For this review, take the finished solid that the model builds, in its own axes (mm). A direction names the side the tool comes from. Round coordinates to 2 decimals unless told otherwise and drop trailing zeros. Write each loop counter-clockwise with the first axis right and the second up, starting at its lowest first coordinate (ties: lowest second). Pieces come first, ordered by that corner, then holes. Notation, with made-up numbers: (25.5, 67.5) - (63.5, 67.5) arc R16 cw to (63.5, 77.5) - close; hole circle Ø7 at (27, 86.5). An arc over 180 degrees is marked (long way). Answer in a Markdown table with one row per item. Add a question column.
from build123d import *

# Parameters (mm, degrees)
SKETCH_1_R          = 15
EXTRUDE_2_DEPTH     = 28
SKETCH_3_R          = 1.5
CUT_EXTRUDE_3_DEPTH = 10
CUT_EXTRUDE_START   = -18
SKETCH_3_2_R        = 1.5
CUT_EXTRUDE_4_DEPTH = 10


with BuildPart() as part:
    # 草图1 → 凸台-拉伸2 (new body)
    with BuildSketch(Plane.XY):
        Circle(SKETCH_1_R)
    extrude(amount=EXTRUDE_2_DEPTH)

    # 草图3 → 切除-拉伸3 (cut)
    with BuildSketch(Plane.XY.offset(28)):
        Circle(SKETCH_3_R)
    extrude(amount=-CUT_EXTRUDE_3_DEPTH, mode=Mode.SUBTRACT)

    # 草图3<2> → 切除-拉伸4 (cut)
    with BuildSketch(Plane.XY.offset(28).offset(CUT_EXTRUDE_START)):
        Circle(SKETCH_3_2_R)
    extrude(amount=-CUT_EXTRUDE_4_DEPTH, mode=Mode.SUBTRACT)


solid = part.part
Q1. Add section D-D on x = -6.5. State the section outline as (y, z) points, then the cut area to 3 significant figures.
Q2. Insertion check: pin 1 Ø1.5 at (y, z) = (1, 5) entering from -X; pin 2 Ø2 at (y, z) = (-11, 22.5) entering from +X. Each pin has a flat end and moves straight along its axis. Give the tip position at first contact, or say it passes through.
Q3. Add section A-A on y = 0. State the section outline as (x, z) points, then the cut area to 3 significant figures.
Q4. Draft analysis for pull direction Y (two halves, no side actions). For faces 4 (the face through (-1.5, 0.07, 5.07)), 5 (the face through (3, 0, 28)), 6 (the face through (-14.985, 0.66, 13.804)), state which applies: released by +Y, released by -Y, zero draft, split by the parting line, or undercut.
Q5. Add section B-B on z = 7.5. State the section outline as (x, y) points.
Q6. To check wall thickness, follow probe 1 along Y at (x, z) = (0, 3); probe 2 along Y at (x, z) = (1.25, 5.25); probe 3 along Y at (x, z) = (9, 20.5). State the ranges of each line that lie inside material, in increasing order.
Q7. Tool access review of faces 1 (the face through (0, 0, 10)), 2 (the face through (0, 0, 18)), 3 (the face through (3, 0, 0)): name each direction out of +Z, -Z, +X, -X, +Y, -Y from which nothing blocks a thin tool from reaching the whole face with its end or side.
Answer sheet:
| question | item | result |
|---|---|---|
| 1 | outline | (-13.52, 0) - (13.52, 0) - (13.52, 28) - (-13.52, 28) - close |
| 1 | area | 757 mm² |
| 2 | pin 1 | stops at x = -15 |
| 2 | pin 2 | stops at x = 11.18 |
| 3 | outline | (-15, 0) - (-1.5, 0) - (-1.5, 10) - (1.5, 10) - (1.5, 0) - (15, 0) - (15, 28) - (1.5, 28) - (1.5, 18) - (-1.5, 18) - (-1.5, 28) - (-15, 28) - close |
| 3 | area | 780 mm² |
| 4 | face 4 | undercut |
| 4 | face 5 | zero draft |
| 4 | face 6 | split by the parting line |
| 5 | outline | circle Ø30 at (0, 0); hole circle Ø3 at (0, 0) |
| 6 | probe 1 | y = -15 to -1.5, 1.5 to 15 |
| 6 | probe 2 | y = -14.95 to -0.83, 0.83 to 14.95 |
| 6 | probe 3 | y = -12 to 12 |
| 7 | face 1 | -Z |
| 7 | face 2 | +Z |
| 7 | face 3 | -Z, +X, -X, +Y, -Y |
